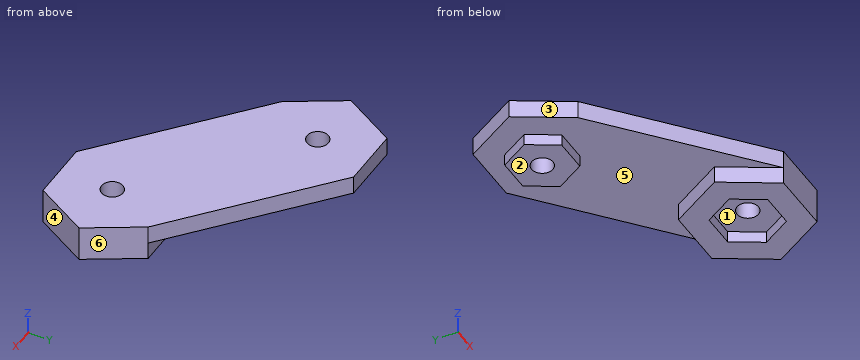
Autodesk Inventor part; units mm, degrees
ref_plane "YZ Plane" through (0, 0, 0) normal (1, 0, 0) x (0, 1, 0)
ref_plane "XZ Plane" through (0, 0, 0) normal (0, 1, 0) x (-1, 0, 0)
ref_plane "XY Plane" through (0, 0, 0) normal (0, 0, 1) x (1, 0, 0)
sketch "Sketch1" plane through (0, 0, 0) normal (0, 0, 1) x (1, 0, 0)
  circle A0 centre (0, 0) radius 12 construction
  line L0 (-68.1273, 0) -> (-34.0637, 59)
  line L1 (-34.0637, 59) -> (34.0637, 59)
  line L2 (34.0637, 59) -> (68.1273, 0)
  line L3 (68.1273, 0) -> (34.0637, -59)
  line L4 (34.0637, -59) -> (-34.0637, -59)
  line L5 (-34.0637, -59) -> (-68.1273, 0)
  dimension "d0" = 24
  dimension "d1" = 118
extrude "Extrusion1" add sketch "Sketch1" along normal blind 40
sketch "Sketch2" plane through (0, 0, 0) normal (0, 0, -1) x (-1, 0, 0)
  line L0 (38.1051, 0) -> (19.0526, -33)
  line L1 (19.0526, -33) -> (-19.0526, -33)
  line L2 (-19.0526, -33) -> (-38.1051, 0)
  line L3 (-38.1051, 0) -> (-19.0526, 33)
  line L4 (-19.0526, 33) -> (19.0526, 33)
  line L5 (19.0526, 33) -> (38.1051, 0)
  circle A0 centre (0, 0) radius 12
  dimension "d4" = 24
  dimension "d5" = 66
extrude "Extrusion2" cut sketch "Sketch2" against normal blind 13 contours L0 L1 L2 L3 L4 L5 | A0
sketch "Sketch3" plane through (0, 0, 40) normal (0, 0, 1) x (1, 0, 0)
  line L0 (-34.0637, -59) -> (34.0637, -59)
  line L1 (-34.0637, -59) -> (-199.0637, 81)
  line L2 (34.0637, 59) -> (-34.0637, 59)
  line L3 (34.0637, 59) -> (-130.9363, 199)
  line L4 (-68.1273, 0) -> (-34.0637, -59)
  line L5 (-34.0637, 59) -> (-68.1273, 0)
  line L6 (-130.9363, 199) -> (-96.8727, 140)
  line L7 (-96.8727, 140) -> (-130.9363, 81)
  line L8 (-130.9363, 81) -> (-199.0637, 81)
  line L9 (-199.0637, 81) -> (-233.1273, 140)
  line L10 (-233.1273, 140) -> (-199.0637, 199)
  line L11 (-199.0637, 199) -> (-130.9363, 199)
  point P0 (0, 0)
  point P1 (-165, 140)
  dimension "d9" = 165
  dimension "d21" = 140
  dimension "d22" = 118
extrude "Extrusion3" add sketch "Sketch3" against normal blind 20.5
sketch "Sketch4" plane through (0, 0, 13) normal (0, 0, -1) x (-1, 0, 0)
  circle A0 centre (0, 0) radius 12
  dimension "d12" = 24
extrude "Extrusion4" cut sketch "Sketch4" against normal through all
sketch "Sketch5" plane through (0, 0, 19.5) normal (0, 0, -1) x (-1, 0, 0)
  line L0 (199.0637, 199) -> (130.9363, 199)
  line L1 (201.9504, 140) -> (183.4752, 108)
  line L2 (183.4752, 108) -> (146.5248, 108)
  line L3 (146.5248, 108) -> (128.0496, 140)
  line L4 (128.0496, 140) -> (146.5248, 172)
  line L5 (146.5248, 172) -> (183.4752, 172)
  line L6 (183.4752, 172) -> (201.9504, 140)
  point P0 (0, 0)
  point P1 (165, 140)
  point P2 (165, 199)
  point P3 (233.1273, 140)
  dimension "d15" = 64
extrude "Extrusion5" add sketch "Sketch5" along normal blind 13
sketch "Sketch6" plane through (0, 0, 6.5) normal (0, 0, -1) x (-1, 0, 0)
  circle A0 centre (165, 140) radius 12
  line L0 (183.4752, 172) -> (146.5248, 172)
  point P0 (0, 0)
  point P1 (201.9504, 140)
  point P2 (165, 172)
  dimension "d18" = 24
extrude "Extrusion6" cut sketch "Sketch6" against normal through all
properties part number "HA10" material "ABS Plastic"
Source: CAD feature listing. Evaluate the final solid. Frame: model axes, mm. Face numbers are marked on the shaded views. A direction names the side the tool comes from. Round coordinates to 2 decimals unless told otherwise and drop trailing zeros. Order: outer loops, then holes, each group sorted by start corner. A loop starts at its lowest first (then second) coordinate and runs counter-clockwise, first axis right, second up. Notation, with made-up numbers: (29, 67) - (44, 67) arc R25 ccw to (44, 99) - close; hole circle Ø8 at (8, -33.5). An arc over 180 degrees is marked (long way). Use a Markdown table: item, result. Add a question column.
1. Set-up query: the marked faces 5 and 6. Return all of +Z, -Z, +X, -X, +Y, -Y with unobstructed straight access to the full face (end or side cutting, diameter ignored); none if empty.
2. Section query B-B (x = 0). Return the cut outline in (y, z), then the cut area to 3 significant figures.
3. Mould query, pull axis X, two halves, no side actions, for the marked faces 1, 2, 3 and 4. Classes: +X half, -X half, draft (parallel to the pull), parting line (faces both ways), or undercut.
4. Line query: probe 1 along Y at (x, z) = (8, 3); probe 2 along Z at (x, y) = (-220, 162.5); probe 3 along Y at (x, z) = (-165, 27). Output: solid intervals per line, ascending.
5. First-contact query: pin 1 (14.5 mm diameter, centred on x = -165, y = 140, fed in from -Z); pin 2 (5 mm diameter, centred on x = -168.5, z = 5.5, fed in from -Y); pin 3 (1 mm diameter, centred on x = -26.5, z = 10.5, fed in from +Y); pin 4 (4 mm diameter, centred on x = -22.5, y = -26, fed in from -Z). Flat tips, straight axial feed; report the tip coordinate or a pass-through.
6. Section query A-A (z = 31.5). Return the cut outline in (x, y), then the cut area to 3 significant figures.
7. Section query C-C (y = 161). Return the cut outline in (x, z), then the cut area to 3 significant figures.
8. Section query D-D (x = -165). Return the cut outline in (y, z).
Derived:
| question | item | result |
|---|---|---|
| 1 | face 5 | -Z |
| 1 | face 6 | +Z, -Z, +X, +Y |
| 2 | outline | (-59, 0) - (-33, 0) - (-33, 13) - (-12, 13) - (-12, 40) - (-59, 40) - close; (12, 13) - (33, 13) - (33, 0) - (59, 0) - (59, 19.5) - (87.9, 19.5) - (87.9, 40) - (12, 40) - close |
| 2 | area | 3,810 mm2 |
| 3 | face 1 | undercut |
| 3 | face 2 | draft |
| 3 | face 3 | -X half |
| 3 | face 4 | +X half |
| 4 | probe 1 | -59 to -33, 33 to 59 |
| 4 | probe 2 | 19.5 to 40 |
| 4 | probe 3 | 52.1 to 128, 152 to 199 |
| 5 | pin 1 | through |
| 5 | pin 2 | y = 108 |
| 5 | pin 3 | y = 59 |
| 5 | pin 4 | z = 0 |
| 6 | outline | (-233.13, 140) - (-199.06, 81) - (-34.06, -59) - (34.06, -59) - (68.13, 0) - (34.06, 59) - (-130.94, 199) - (-199.06, 199) - close; hole circle Ø24 at (-165, 140); hole circle Ø24 at (0, 0) |
| 6 | area | 40,200 mm2 |
| 7 | outline | (-221, 19.5) - (-189.83, 19.5) - (-189.83, 6.5) - (-140.17, 6.5) - (-140.17, 19.5) - (-86.15, 19.5) - (-86.15, 40) - (-221, 40) - close |
| 7 | area | 3,410 mm2 |
| 8 | outline | (52.1, 19.5) - (108, 19.5) - (108, 6.5) - (128, 6.5) - (128, 40) - (52.1, 40) - close; (152, 6.5) - (172, 6.5) - (172, 19.5) - (199, 19.5) - (199, 40) - (152, 40) - close |
